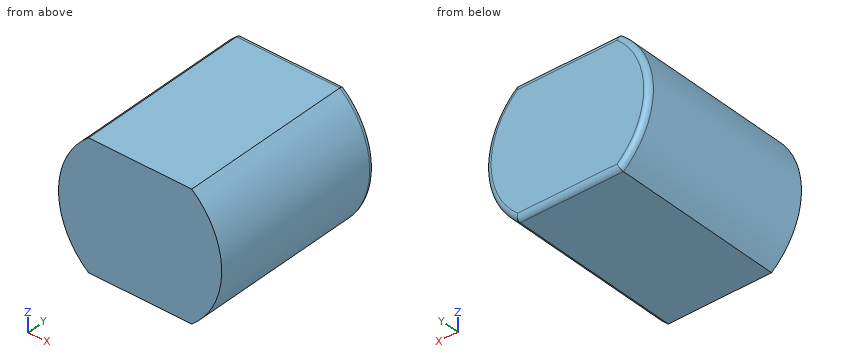
```python
from build123d import *

# Parameters (mm, degrees)
SALIENTE_EXTRUIR1_DEPTH = 17
REDONDEO1_R             = 0.5


with BuildPart() as part:
    # Croquis1 → Saliente-Extruir1 (new body)
    with BuildSketch(Plane(origin=(0, 0, 0), x_dir=(1, 0, 0), z_dir=(0, 1, 0))):
        with BuildLine():
            Line((-4.905354218, -6), (4.905354218, -6))
            ThreePointArc((4.905354218, -6), (7.75, 0), (4.905354218, 6))
            Line((4.905354218, 6), (-4.905354218, 6))
            ThreePointArc((-4.905354218, 6), (-7.75, 0), (-4.905354218, -6))
        make_face()
    extrude(amount=SALIENTE_EXTRUIR1_DEPTH)

    # Redondeo1
    redondeo1_edges = [part.edges().sort_by_distance(p)[0] for p in [
        (-7.75, 17, 0),
        (0, 17, 6),
        (7.75, 17, 0),
        (0, 17, -6),
    ]]
    fillet(redondeo1_edges, radius=REDONDEO1_R)


solid = part.part
```
Input: part model. Units: mm. Frame: model coordinates. Round coordinates to 2 decimals unless told otherwise and drop trailing zeros. Write each loop counter-clockwise with the first axis right and the second up, starting at its lowest first coordinate (ties: lowest second). Pieces come first, ordered by that corner, then holes. Notation, with made-up numbers: (66.25, 27.25) - (91.25, 27.25) arc R20 cw to (91.25, 38.25) - close; hole circle Ø8 at (-6, -19.5). An arc over 180 degrees is marked (long way). Write item = value, one per line.
(1) Section query A-A on y = 4.75. Output: boundary loops of the cut face in (x, z).
Geometry check:
outline = (-4.91, -6) - (4.91, -6) arc R7.75 ccw to (4.91, 6) - (-4.91, 6) arc R7.75 ccw to start
(2) Contact query for flat-ended pins moving along their axis: pin 1 Ø2 at (y, z) = (10, 3) entering from -X; pin 2 Ø5 at (y, z) = (3, -5) entering from -X; pin 3 Ø3 at (y, z) = (12, 3) entering from +X. Output: stop coordinate, or through.
Geometry check:
pin_1 = -7.49
pin_2 = -7.34
pin_3 = 7.6
(3) Material intervals for probe 1 along X at (y, z) = (15, -0.25); probe 2 along Z at (x, y) = (-7, 7.5); probe 3 along X at (y, z) = (2, -4), sorted ascending.
Geometry check:
probe_1 = -7.75 to 7.75
probe_2 = -3.33 to 3.33
probe_3 = -6.64 to 6.64
